Drawing for the job (mm, zero at the part's lowest x, y, z). A direction names the side the tool comes from. Round coordinates to 2 decimals unless told otherwise and drop trailing zeros. Write each loop counter-clockwise with the first axis right and the second up, starting at its lowest first coordinate (ties: lowest second). Pieces come first, ordered by that corner, then holes.
Item 1: Band-saw the part on A-A, the plane z = 1.65. Count the separate pieces of the cut face and the enclosed holes in it, then the cut area to 3 significant figures.
Item 2: 3-axis set-ups, long thin cutter, end or side, ignore diameter. For the marked faces 1, 2 and 3: which of +Z, -Z, +X, -X, +Y, -Y reach the whole face in a straight line?
Item 3: Band-saw the part on C-C, the plane x = 20. Write the cut outline in (y, z).
Item 4: Wall check: probe 1 along Y at (x, z) = (13, 2.1); probe 2 along X at (y, z) = (48, 2.3); probe 3 along Y at (x, z) = (21.5, 1.6). Give the ranges that are in metal, low to high.
Item 5: Band-saw the part on B-B, the plane y = 52. Write the cut outline in (x, z), then the cut area to 3 significant figures.
Item 6: Drop flat-ended pins along their axis: pin 1 Ø3 at (x, z) = (5, 1) entering from +Y; pin 2 Ø6 at (x, y) = (17.5, 14.5) entering from -Z; pin 3 Ø3 at (y, z) = (63.5, 3.5) entering from -X. Give the stop position or say it passes through.
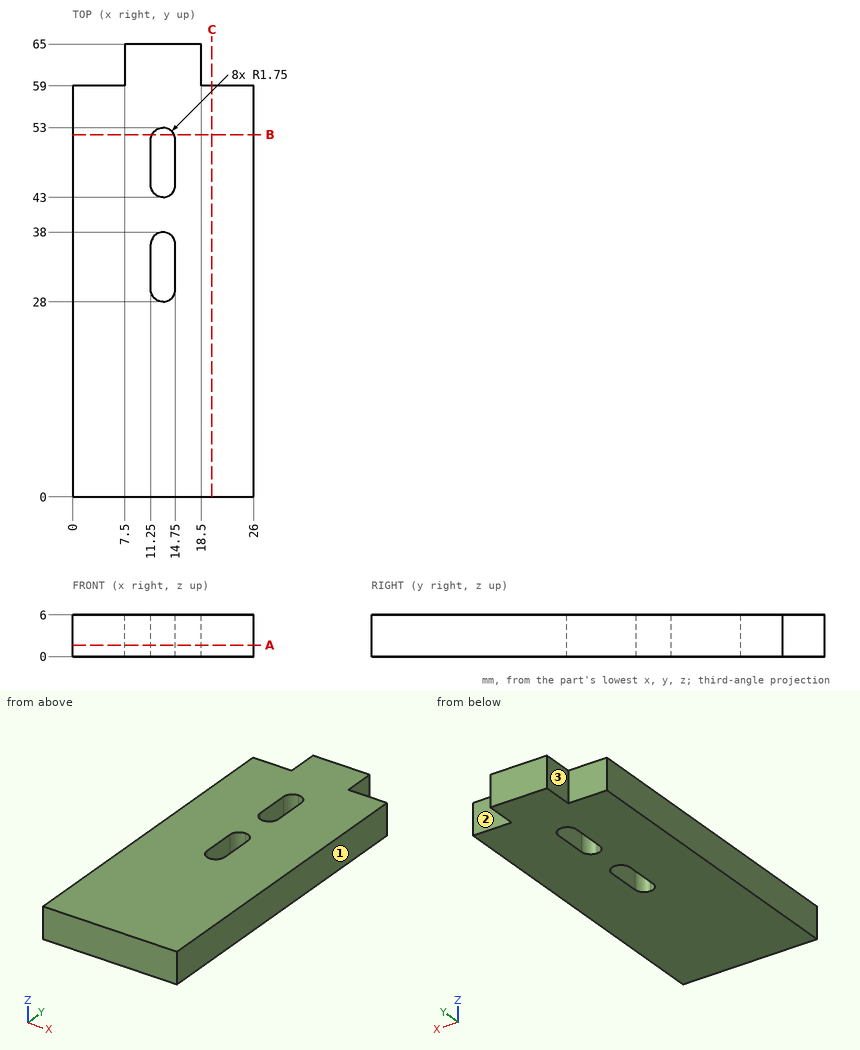
Results:
1. separate pieces: 1
1. enclosed holes: 2
1. area: 1,540 mm2
2. face 1: +Z, -Z, +X, +Y, -Y
2. face 2: +Z, -Z, +X, +Y
2. face 3: +Z, -Z, -X, +Y
3. outline: (0, 0) - (59, 0) - (59, 6) - (0, 6) - close
4. probe 1: y = 0 to 28, 38 to 43, 53 to 65
4. probe 2: x = 0 to 11.25, 14.75 to 26
4. probe 3: y = 0 to 59
5. outline: (0, 0) - (11.42, 0) - (11.42, 6) - (0, 6) - close; (14.58, 0) - (26, 0) - (26, 6) - (14.58, 6) - close
5. area: 137 mm2
6. pin 1: stops at y = 59
6. pin 2: stops at z = 0
6. pin 3: stops at x = 7.5
